Drawing for the job (mm, zero at the part's lowest x, y, z). A direction names the side the tool comes from. Round coordinates to 2 decimals unless told otherwise and drop trailing zeros. Write each loop counter-clockwise with the first axis right and the second up, starting at its lowest first coordinate (ties: lowest second). Pieces come first, ordered by that corner, then holes. Notation, with made-up numbers: M -30,-23.75 L -1,-23.75 A17 cw -1,-5.75 Z; hole C 8,84.25 d9. An arc over 180 degrees is marked long. Use a Markdown table: item, result. Add a question column.
1) Slice it at C-C on y = 26. Write the cut outline in (x, z).
2) Slice it at A-A on x = 108. Write the cut outline in (y, z).
3) Slice it at D-D on z = 25.65. Write the cut outline in (x, y).
4) Drop flat-ended pins along their axis: P1, Ø3.5, axis at x = 68.35, z = 56.65, coming from the -Y side; P2, Ø3.5, axis at x = 20.65, z = 25.65, coming from the +Y side; P3, Ø4, axis at y = 5, z = 137.82, coming from the +X side. Give the stop position or say it passes through.
5) Two-plate mould, pull along X, no slides. Class the marked faces 1, 2, 3 and 4: released by +X, released by -X, zero draft, split by the parting line, or undercut.
6) Which spindle directions (+Z, -Z, +X, -X, +Y, -Y) get a long thin tool onto all of the face, cutting with end or side? Do the marked faces 5, 6 and 7. Say none if no direction does.
7) Wall check: probe 1 along Z at (x, y) = (68.35, 15.75); probe 2 along X at (y, z) = (24, 79.5); probe 3 along X at (y, z) = (9, 61). Give the ranges that are in metal, low to high.
8) Slice it at B-B on z = 73.95. Write the cut outline in (x, y).
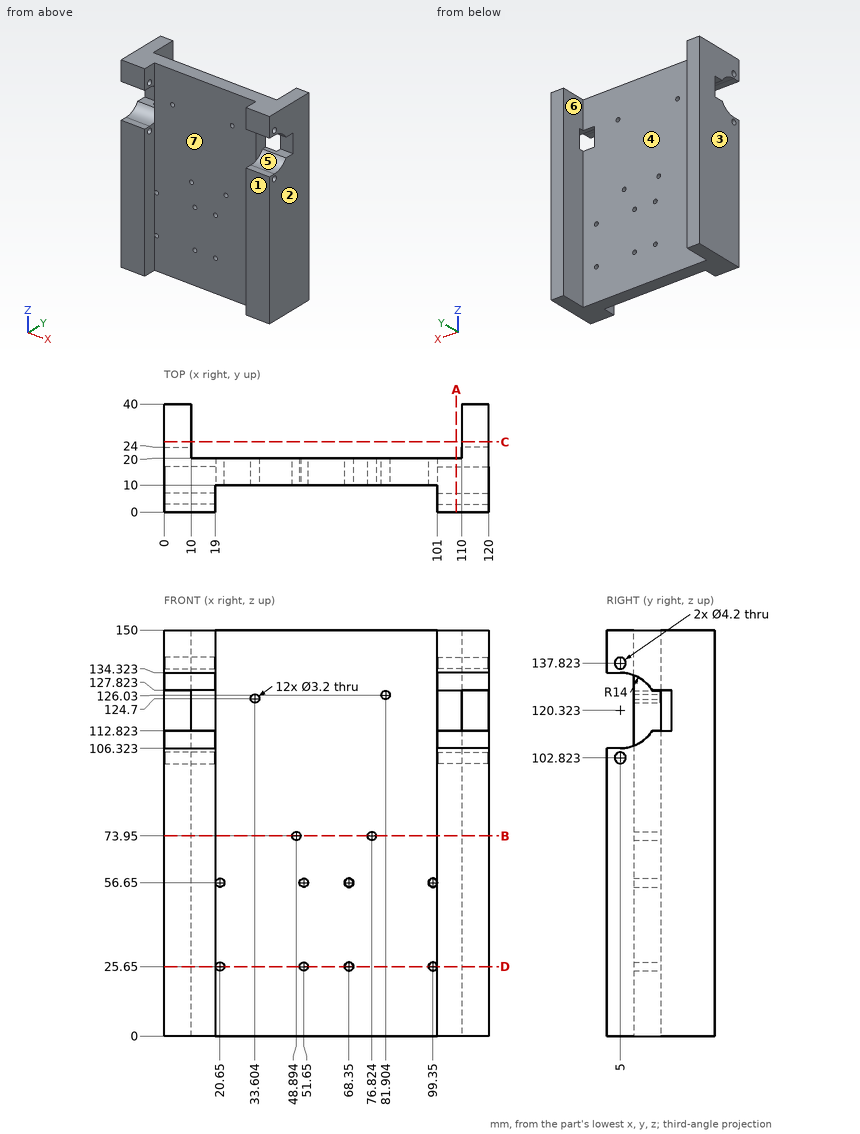
Entries:
| question | item | result |
|---|---|---|
| 1 | outline | M 0,0 L 10,0 L 10,150 L 0,150 Z; M 110,0 L 120,0 L 120,150 L 110,150 Z |
| 2 | outline | M 0,0 L 20,0 L 20,112.82 L 16.82,112.82 A14 cw 5,106.32 L 0,106.32 Z; M 0,134.32 L 5,134.32 A14 cw 16.82,127.82 L 20,127.82 L 20,150 L 0,150 Z; hole C 5,102.82 d4.2; hole C 5,137.82 d4.2 |
| 3 | outline | M 0,0 L 19,0 L 19,10 L 19.05,10 L 19.05,20 L 10,20 L 10,40 L 0,40 Z; M 22.25,10 L 50.05,10 L 50.05,20 L 22.25,20 Z; M 53.25,10 L 66.75,10 L 66.75,20 L 53.25,20 Z; M 69.95,10 L 97.75,10 L 97.75,20 L 69.95,20 Z; M 100.95,10 L 101,10 L 101,0 L 120,0 L 120,40 L 110,40 L 110,20 L 100.95,20 Z |
| 4 | P1 | stops at y = 10 |
| 4 | P2 | stops at y = 20 |
| 4 | P3 | passes through |
| 5 | face 1 | zero draft |
| 5 | face 2 | released by +X |
| 5 | face 3 | released by -X |
| 5 | face 4 | undercut |
| 6 | face 5 | +X, -Y |
| 6 | face 6 | +Z, -Z, +Y |
| 6 | face 7 | +Z, -Z, -Y |
| 7 | probe 1 | z = 0 to 24.05, 27.25 to 55.05, 58.25 to 150 |
| 7 | probe 2 | x = 0 to 10, 110 to 120 |
| 7 | probe 3 | x = 0 to 19, 101 to 120 |
| 8 | outline | M 0,0 L 19,0 L 19,10 L 47.29,10 L 47.29,20 L 10,20 L 10,40 L 0,40 Z; M 50.49,10 L 75.22,10 L 75.22,20 L 50.49,20 Z; M 78.42,10 L 101,10 L 101,0 L 120,0 L 120,40 L 110,40 L 110,20 L 78.42,20 Z |
